Source: CAD feature listing. Evaluate the final solid. Frame: model axes, mm. Face numbers are marked on the shaded views. A direction names the side the tool comes from. Round coordinates to 2 decimals unless told otherwise and drop trailing zeros. Write each loop counter-clockwise with the first axis right and the second up, starting at its lowest first coordinate (ties: lowest second). Pieces come first, ordered by that corner, then holes. Notation, with made-up numbers: (41.5, -5.75) -> (87.5, -5.75) arc R19 cw to (87.5, 6.25) -> close; hole circle Ø1 at (88.25, 45). An arc over 180 degrees is marked (long way). Put each result on its own line as item: value.
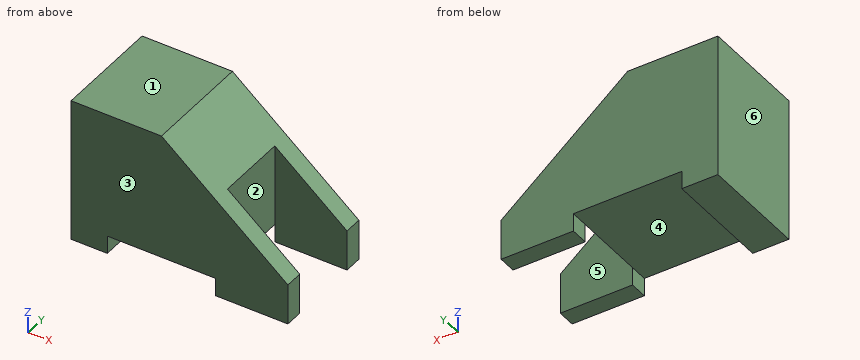
```python
from build123d import *

# Parameters (mm, degrees)
F1_DEPTH = 7.5
F2_W     = 35.456628
F2_H     = 10
F3_DEPTH = 20.001


with BuildPart() as f1:
    # F0 (on Front) → F1 (new body, symmetric)
    with BuildSketch(Plane.XZ):
        Polygon((0, 20), (0, 0), (5, 0), (5, 2.5), (20, 2.5), (20, 0), (30, 0), (30, 5.639098), (12.5, 20), align=None)
    extrude(amount=F1_DEPTH, both=True)

    # F2 (on face) → F3 (cut, through all)
    with BuildSketch(Plane(origin=(0, 0, 0), x_dir=(1, 0, 0), z_dir=(0, 0, -1))):
        with Locations((37.728314, 0)):
            Rectangle(F2_W, F2_H)
    extrude(amount=-F3_DEPTH, mode=Mode.SUBTRACT)


solid = f1.part
```
Q1. Material intervals for line 1 (Y direction, x = 23.75, z = 7.25); line 2 (X direction, y = -3.5, z = 7.5); line 3 (X direction, y = 4.75, z = 1.5), sorted ascending. Write a range as [from, to].
Ans:
line 1: y = [-7.5, -5], [5, 7.5]
line 2: x = [0, 20]
line 3: x = [0, 5]
Q2. Draft query along Y for the marked faces 1, 2 and 3. Return one class per face: +Y half, -Y half, draft (parallel to the pull), parting line (faces both ways), or undercut.
Ans:
face 1: draft
face 2: undercut
face 3: -Y half
Q3. Pin query (flat end, axial travel): pin 1 (1 mm diameter, centred on y = -2, z = 16, fed in from +X); pin 2 (1.5 mm diameter, centred on y = 1.5, z = 10.5, fed in from +X); pin 3 (4.5 mm diameter, centred on x = 10, y = 2.5, fed in from -Z). Return the tip coordinate at first contact, or that it passes through.
Ans:
pin 1: stops at x = 17.98
pin 2: stops at x = 20
pin 3: stops at z = 2.5
Q4. Cut plane A-A on y = 0.75. Output: boundary loops of the cut face in (x, z).
Ans:
outline: (0, 0) -> (5, 0) -> (5, 2.5) -> (20, 2.5) -> (20, 13.85) -> (12.5, 20) -> (0, 20) -> close
Q5. Cut plane C-C on x = 25.5. Output: boundary loops of the cut face in (y, z).
Ans:
outline: (-7.5, 0) -> (-5, 0) -> (-5, 9.33) -> (-7.5, 9.33) -> close; (5, 0) -> (7.5, 0) -> (7.5, 9.33) -> (5, 9.33) -> close
Q6. Cut plane B-B on z = 5. Output: boundary loops of the cut face in (x, y), and give its area (3 significant figures).
Ans:
outline: (0, -7.5) -> (30, -7.5) -> (30, -5) -> (20, -5) -> (20, 5) -> (30, 5) -> (30, 7.5) -> (0, 7.5) -> close
area: 350 mm^2
Q7. Cut plane D-D on y = 5.75. Output: boundary loops of the cut face in (x, z).
Ans:
outline: (0, 0) -> (5, 0) -> (5, 2.5) -> (20, 2.5) -> (20, 0) -> (30, 0) -> (30, 5.64) -> (12.5, 20) -> (0, 20) -> close
Q8. Reachability of the marked faces 4, 5 and 6 from +Z, -Z, +X, -X, +Y, -Y: full face, straight path, thin tool, end or side. Return the list, or none.
Ans:
face 4: -Z, +Y, -Y
face 5: +Z, -Z, +X
face 6: +Z, -Z, -X, +Y, -Y
